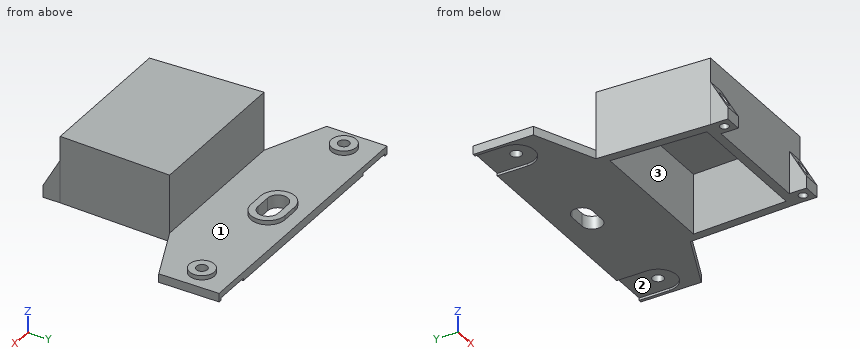
```python
from build123d import *

# Parameters (mm, degrees)
MAIN_BODY_DEPTH                    = 6.35
POCKET_OUTER_SURFACE_DEPTH         = 43.18
POCKET_INSIDE_DEPTH                = 44.45
SKETCH8_W                          = 12.7
SKETCH8_H                          = 31.75
BOTTOM_SCREW_MOUNT_DEPTH           = 12.7
BOTTOM_SCREW_MOUNT_EXTRUSION_DEPTH = 218.712414724
LIGHT_SOCKETS_DEPTH                = 184.078329957
LIGHT_SOCKETS_DEPTH_BACK           = 6.35
SKETCH17_R                         = 4.064
SKETCH18_R                         = 9.144
LIGHT_LIP_LINERS_DEPTH             = 3.175
LIGHT_LIP_SOCKETS_REACH            = 185.078
SKETCH17_2_R                       = 4.064
TAB_SLOTS_DEPTH                    = 1.778
F_1_4_0_25_DIAMETER_HOLE1_D        = 6.35


# Sheet-metal steps are written as plain solids
with BuildPart() as part:
    # Sketch1 → Main Body (new body)
    with BuildSketch(Plane.XY):
        Polygon((-53.975, 0), (53.975, 0), (57.15, 82.55), (101.6, 101.6), (101.6, 146.05), (-101.6, 146.05), (-101.6, 101.6), (-57.15, 82.55), align=None)
    extrude(amount=-MAIN_BODY_DEPTH)

    # Sketch6 → Pocket-Outer Surface (add)
    with BuildSketch(Plane.XY):
        Polygon((53.975, 0), (-53.975, 0), (-57.15, 82.55), (57.15, 82.55), align=None)
    extrude(amount=POCKET_OUTER_SURFACE_DEPTH)

    # Sketch7 → Pocket-Inside (cut)
    with BuildSketch(Plane(origin=(0, 0, -6.35), x_dir=(-1, 0, 0), z_dir=(0, 0, -1))):
        Polygon((-50.551074221, 76.2), (-47.864535759, 6.35), (47.864535759, 6.35), (50.551074221, 76.2), align=None)
    extrude(amount=-POCKET_INSIDE_DEPTH, mode=Mode.SUBTRACT)

    # Sketch8 → Bottom Screw Mount (add)
    with BuildSketch(Plane.XZ):
        with Locations((-47.625, 9.525)):
            Rectangle(SKETCH8_W, SKETCH8_H)
    bottom_screw_mount = extrude(amount=BOTTOM_SCREW_MOUNT_DEPTH)

    # Sketch9 → Bottom Screw Mount Extrusion (cut, through all)
    with BuildSketch(Plane.ZY.offset(53.975)):
        Polygon((2.54, -12.7), (25.4, -12.7), (25.4, 0), align=None)
    bottom_screw_mount_extrusion = extrude(amount=-BOTTOM_SCREW_MOUNT_EXTRUSION_DEPTH, mode=Mode.SUBTRACT)

    # Left Bottom Screw Mount: Bottom Screw Mount, Bottom Screw Mount Extrusion across plane
    add(bottom_screw_mount.mirror(Plane(origin=(0, 0, 0), x_dir=(0, 0, 1), z_dir=(1, 0, 0))))
    add(bottom_screw_mount_extrusion.mirror(Plane(origin=(0, 0, 0), x_dir=(0, 0, 1), z_dir=(1, 0, 0))), mode=Mode.SUBTRACT)

    # Sketch17 → Light Sockets (cut, two sides: drawn at the far end of the back side and taken through both)
    with BuildSketch(Plane.XY.offset(-LIGHT_SOCKETS_DEPTH_BACK)):
        with Locations((85.852, 123.825)):
            Circle(SKETCH17_R)
        with Locations((-85.852, 123.825)):
            Circle(SKETCH17_R)
        with BuildLine():
            Line((-5.969, 131.318), (5.969, 131.318))
            ThreePointArc((5.969, 131.318), (13.462, 123.825), (5.969, 116.332))
            Line((5.969, 116.332), (-5.969, 116.332))
            ThreePointArc((-5.969, 116.332), (-13.462, 123.825), (-5.969, 131.318))
        make_face()
    extrude(amount=LIGHT_SOCKETS_DEPTH + LIGHT_SOCKETS_DEPTH_BACK, mode=Mode.SUBTRACT)

    # Sketch18 → Light Lip Liners (add)
    with BuildSketch(Plane.XY):
        with Locations((-85.852, 123.825)):
            Circle(SKETCH18_R)
        with Locations((85.852, 123.825)):
            Circle(SKETCH18_R)
        with BuildLine():
            Line((5.969, 136.398), (-5.969, 136.398))
            ThreePointArc((-5.969, 136.398), (-18.542, 123.825), (-5.969, 111.252))
            Line((-5.969, 111.252), (5.969, 111.252))
            ThreePointArc((5.969, 111.252), (18.542, 123.825), (5.969, 136.398))
        make_face()
    extrude(amount=LIGHT_LIP_LINERS_DEPTH)

    # Sketch17<2> → Light Lip Sockets (cut, up to next)
    with BuildSketch(Plane.XY, mode=Mode.PRIVATE) as light_lip_sockets_sk1:
        with Locations((85.852, 123.825)):
            Circle(SKETCH17_2_R)
    light_lip_sockets_tool1 = extrude(light_lip_sockets_sk1.sketch, amount=LIGHT_LIP_SOCKETS_REACH, mode=Mode.PRIVATE) & part.part
    # Sketch17<2> → Light Lip Sockets (cut, up to next)
    with BuildSketch(Plane.XY, mode=Mode.PRIVATE) as light_lip_sockets_sk2:
        with Locations((-85.852, 123.825)):
            Circle(SKETCH17_2_R)
    light_lip_sockets_tool2 = extrude(light_lip_sockets_sk2.sketch, amount=LIGHT_LIP_SOCKETS_REACH, mode=Mode.PRIVATE) & part.part
    # Sketch17<2> → Light Lip Sockets (cut, up to next)
    with BuildSketch(Plane.XY, mode=Mode.PRIVATE) as light_lip_sockets_sk3:
        with BuildLine():
            Line((-5.969, 131.318), (5.969, 131.318))
            ThreePointArc((5.969, 131.318), (13.462, 123.825), (5.969, 116.332))
            Line((5.969, 116.332), (-5.969, 116.332))
            ThreePointArc((-5.969, 116.332), (-13.462, 123.825), (-5.969, 131.318))
        make_face()
    light_lip_sockets_tool3 = extrude(light_lip_sockets_sk3.sketch, amount=LIGHT_LIP_SOCKETS_REACH, mode=Mode.PRIVATE) & part.part
    add(light_lip_sockets_tool1.solids().sort_by_distance((85.852, 123.825, 0))[0], mode=Mode.SUBTRACT)
    add(light_lip_sockets_tool2.solids().sort_by_distance((-85.852, 123.825, 0))[0], mode=Mode.SUBTRACT)
    add(light_lip_sockets_tool3.solids().sort_by_distance((0, 123.825, 0))[0], mode=Mode.SUBTRACT)

    # Sketch19 → Tab Slots (cut)
    with BuildSketch(Plane(origin=(0, 0, -6.35), x_dir=(-1, 0, 0), z_dir=(0, 0, -1))):
        with BuildLine():
            Line((72.263, 146.05), (72.263, 123.825))
            ThreePointArc((72.263, 123.825), (85.852, 110.236), (99.441, 123.825))
            Line((99.441, 123.825), (99.441, 146.05))
            Line((99.441, 146.05), (72.263, 146.05))
        make_face()
    tab_slots = extrude(amount=-TAB_SLOTS_DEPTH, mode=Mode.SUBTRACT)

    # Mirror3: Tab Slots across plane
    add(tab_slots.mirror(Plane(origin=(0, 0, 0), x_dir=(0, 0, 1), z_dir=(1, 0, 0))), mode=Mode.SUBTRACT)

    # 1/4 (0.25) Diameter Hole1 (through all)
    with Locations(Plane(origin=(0, 0, -6.35), x_dir=(-1, 0, 0), z_dir=(0, 0, -1))):
        with Locations((-47.625, -6.35), (47.625, -6.35)):
            Hole(F_1_4_0_25_DIAMETER_HOLE1_D / 2)


solid = part.part
```
Here's how the part is built. I have some questions about the finished solid (model axes, mm). Face numbers are marked on the shaded views. A direction names the side the tool comes from. Give positions to 0.01 mm unless a question says otherwise; leave off trailing zeros. Write each loop counter-clockwise with the first axis right and the second up, starting at its lowest first coordinate (ties: lowest second). Pieces come first, ordered by that corner, then holes. Notation, with made-up numbers: (15, 66.25) -> (51, 66.25) arc R22 ccw to (51, 105.25) -> close; hole circle Ø3 at (8.25, -31). An arc over 180 degrees is marked (long way). Use one line per item in the form item = value.
1) If I drill on L1, parallel to X at y = -6.35, z = 0.75 (3 decimals); L2, parallel to Y at x = -24.5, z = 6.5; L3, parallel to Z at x = 69.5, y = 111, over which ranges is the centre line in solid material (lowest first)? Write a range as [from, to].
Verdict:
L1 = [-53.975, -50.8], [-44.45, -41.275], [41.275, 44.45], [50.8, 53.975]
L2 = [0, 6.35], [76.2, 82.55]
L3 = [-6.35, 0]
2) I'm going to push flat-ended pins straight in: pin 1 (1.5 mm diameter, centred on x = 50, z = 5, fed in from -Y); pin 2 (20 mm diameter, centred on x = -5, y = 128.5, fed in from +Z) (3 decimals); pin 3 (1.5 mm diameter, centred on x = 16.5, z = 9, fed in from +Y). Where does each tip first touch, or does it pass through?
Verdict:
pin_1 = -11.75
pin_2 = 3.175
pin_3 = 82.55
3) Suppose I cut it at B-B (z = 5.5). Please give me the cut outline in (x, y) (3 decimals), and give its area (3 significant figures).
Verdict:
outline = (-57.15, 82.55) -> (-53.975, 0) -> (-53.975, -11.056) -> (-41.275, -11.056) -> (-41.275, 0) -> (41.275, 0) -> (41.275, -11.056) -> (53.975, -11.056) -> (53.975, 0) -> (57.15, 82.55) -> close; hole circle Ø6.35 at (-47.625, -6.35); hole (-50.551, 76.2) -> (-47.865, 6.35) -> (47.865, 6.35) -> (50.551, 76.2) -> close; hole circle Ø6.35 at (47.625, -6.35)
area = 2,520 mm2
4) Suppose I cut it at D-D (z = 22). Please give me the cut outline in (x, y) (3 decimals), and give its area (3 significant figures).
Verdict:
outline = (-57.15, 82.55) -> (-53.975, 0) -> (-53.975, -1.889) -> (-41.275, -1.889) -> (-41.275, 0) -> (41.275, 0) -> (41.275, -1.889) -> (53.975, -1.889) -> (53.975, 0) -> (57.15, 82.55) -> close; hole (-50.551, 76.2) -> (-47.865, 6.35) -> (47.865, 6.35) -> (50.551, 76.2) -> close
area = 2,350 mm2
5) Suppose I cut it at A-A (y = -6.35). Please give me the cut outline in (x, z) (3 decimals).
Verdict:
outline = (-53.975, -6.35) -> (-50.8, -6.35) -> (-50.8, 13.97) -> (-53.975, 13.97) -> close; (-44.45, -6.35) -> (-41.275, -6.35) -> (-41.275, 13.97) -> (-44.45, 13.97) -> close; (41.275, -6.35) -> (44.45, -6.35) -> (44.45, 13.97) -> (41.275, 13.97) -> close; (50.8, -6.35) -> (53.975, -6.35) -> (53.975, 13.97) -> (50.8, 13.97) -> close
6) Suppose I cut it at C-C (y = 15.5). Please give me the cut outline in (x, z), and give its area (3 significant figures).
Verdict:
outline = (-54.57, -6.35) -> (-48.22, -6.35) -> (-48.22, 38.1) -> (48.22, 38.1) -> (48.22, -6.35) -> (54.57, -6.35) -> (54.57, 43.18) -> (-54.57, 43.18) -> close
area = 1,120 mm2
7) On a 3-axis mill with a long thin cutter (end or side, diameter ignored), from which of +Z, -Z, +X, -X, +Y, -Y can I reach the whole of each face in a straight line? I mean the marked faces 1, 2 and 3. Say none if no direction works.
Verdict:
face_1 = +Z
face_2 = -Z, +Y
face_3 = -Z
